from build123d import *

# Parameters (mm, degrees)
SKETCH1_W           = 10
SKETCH1_H           = 10
SKETCH1_W_2         = 8
SKETCH1_H_2         = 8
BOSS_EXTRUDE1_DEPTH = 572
SKETCH2_R           = 2.1
CUT_EXTRUDE1_DEPTH  = 116
SKETCH3_R           = 2.1
CUT_EXTRUDE2_DEPTH  = 5
SKETCH5_R           = 2.1
CUT_EXTRUDE3_DEPTH  = 10


with BuildPart() as part:
    # Sketch1 → Boss-Extrude1 (new body)
    with BuildSketch(Plane.XY):
        with Locations((5, 5)):
            Rectangle(SKETCH1_W, SKETCH1_H)
        with Locations((5, 5)):
            Rectangle(SKETCH1_W_2, SKETCH1_H_2, mode=Mode.SUBTRACT)
    extrude(amount=BOSS_EXTRUDE1_DEPTH)

    # Sketch2 → Cut-Extrude1 (cut)
    with BuildSketch(Plane(origin=(0, 10, 0), x_dir=(1, 0, 0), z_dir=(0, 1, 0))):
        with Locations(Location((5, -5, 0), (0, 0, 270))):
            Circle(SKETCH2_R)
        with Locations(Location((5, -15, 0), (0, 0, 270))):
            Circle(SKETCH2_R)
        with Locations(Location((5, -557, 0), (0, 0, 270))):
            Circle(SKETCH2_R)
        with Locations(Location((5, -567, 0), (0, 0, 270))):
            Circle(SKETCH2_R)
    extrude(amount=-CUT_EXTRUDE1_DEPTH, mode=Mode.SUBTRACT)

    # Sketch3 → Cut-Extrude2 (cut)
    with BuildSketch(Plane.XZ):
        with Locations(Location((5, 336, 0), (0, 0, 270))):
            Circle(SKETCH3_R)
        with Locations(Location((5, 236, 0), (0, 0, 270))):
            Circle(SKETCH3_R)
    extrude(amount=-CUT_EXTRUDE2_DEPTH, mode=Mode.SUBTRACT)

    # Sketch5 → Cut-Extrude3 (cut)
    with BuildSketch(Plane(origin=(10, 0, 0), x_dir=(0, 0, -1), z_dir=(1, 0, 0))):
        with Locations(Location((-472, 5, 0), (0, 0, 90))):
            Circle(SKETCH5_R)
        with Locations(Location((-100, 5, 0), (0, 0, 90))):
            Circle(SKETCH5_R)
        with Locations(Location((-286, 5, 0), (0, 0, 90))):
            Circle(SKETCH5_R)
    extrude(amount=-CUT_EXTRUDE3_DEPTH, mode=Mode.SUBTRACT)


solid = part.part
Geometry: final body of the model. Coordinates: model frame, mm. Give positions to 0.01 mm unless a question says otherwise; leave off trailing zeros. Order: outer loops, then holes, each group sorted by start corner. A loop starts at its lowest first (then second) coordinate and runs counter-clockwise, first axis right, second up. Notation, with made-up numbers: (-20, -23) - (-9, -23) arc R27 cw to (-9, 13) - close; hole circle Ø6 at (-17.75, -39). An arc over 180 degrees is marked (long way). Use CSV: the item, a comma, the result in double quotes.
1. Section query A-A (y = 5). Give the number of separate pieces and of enclosed holes in the cut face, plus the area to 3 significant figures.
Answers below:
separate pieces,"8"
enclosed holes,"0"
area,"1,120 mm2"
2. Material intervals for line 1 along Z through (x, y) = (9.6, 5); line 2 along X through (y, z) = (1.75, 234); line 3 along Z through (x, y) = (4, 9.75), sorted ascending. Write a range as from..to.
Answers below:
line 1,"0..97.9, 102.1..283.9, 288.1..469.9, 474.1..572"
line 2,"0..1, 9..10"
line 3,"0..3.15, 6.85..13.15, 16.85..555.15, 558.85..565.15, 568.85..572"
3. Section query B-B (z = 416). Output: boundary loops of the cut face in (x, y).
Answers below:
outline,"(0, 0) - (10, 0) - (10, 10) - (0, 10) - close; hole (1, 1) - (9, 1) - (9, 9) - (1, 9) - close"
